Verification items for the finished model (mm, model axes). Face numbers are marked on the shaded views. A direction names the side the tool comes from. Round coordinates to 2 decimals unless told otherwise and drop trailing zeros. Write each loop counter-clockwise with the first axis right and the second up, starting at its lowest first coordinate (ties: lowest second). Pieces come first, ordered by that corner, then holes. Notation, with made-up numbers: (22, -22) - (49, -22) arc R13 ccw to (49, -15) - close; hole circle Ø8 at (41.25, -23.75). An arc over 180 degrees is marked (long way). Answer as a JSON object with one key per item and string values.
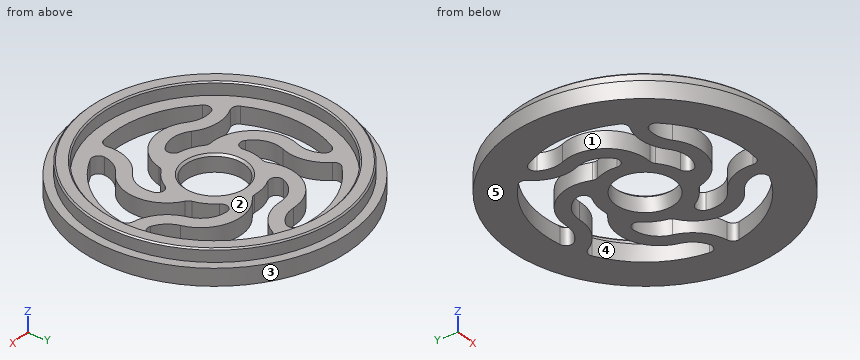
```python
from build123d import *

# Parameters (mm, degrees)
F3_DEPTH = 25.4


with BuildPart() as f1:
    # F0 (on Front) → F1 (revolve)
    with BuildSketch(Plane.XZ):
        Polygon((-25.4, 0), (-5.4737, 0), (-5.4737, 2.794), (-5.8547, 3.175), (-21.3995, 3.175), (-21.3995, 5.334), (-21.6535, 5.588), (-23.5585, 5.588), (-23.8125, 5.334), (-23.8125, 3.175), (-25.4, 3.175), align=None)
    revolve(axis=Axis((0, 0, 7.17671), (0, 0, 1)))

    # F2 (on face) → F3 (cut)
    with BuildSketch(Plane.XY.offset(3.175)):
        with BuildLine():
            ThreePointArc((-7.956627, -0.95471), (-7.931805, 1.142742), (-7.363544, 3.1619))
            ThreePointArc((-7.363544, 3.1619), (-7.260521, 3.657138), (-7.358972, 4.153304))
            ThreePointArc((-7.358972, 4.153304), (-6.561517, 11.480324), (0.065952, 14.704886))
            ThreePointArc((0.065952, 14.704886), (2.327191, 15.1072), (4.180137, 16.464274))
            ThreePointArc((4.180137, 16.464274), (4.415643, 17.713968), (3.449856, 18.541285))
            ThreePointArc((3.449856, 18.541285), (-5.482341, 18.045073), (-13.180977, 13.488609))
            ThreePointArc((-13.180977, 13.488609), (-13.563205, 12.600734), (-13.209763, 11.701011))
            ThreePointArc((-13.209763, 11.701011), (-11.238972, 7.93406), (-11.593134, 3.697492))
            ThreePointArc((-11.593134, 3.697492), (-11.749757, 0.538425), (-10.006841, -2.100984))
            ThreePointArc((-10.006841, -2.100984), (-8.597816, -2.214519), (-7.956627, -0.95471))
        make_face()
        with BuildLine():
            ThreePointArc((-1.55075, -7.862224), (-3.537875, -7.190468), (-5.282606, -6.026065))
            ThreePointArc((-5.282606, -6.026065), (-5.721769, -5.775048), (-6.224075, -5.715357))
            ThreePointArc((-6.224075, -5.715357), (-12.946057, -2.692759), (-13.964798, 4.606784))
            ThreePointArc((-13.964798, 4.606784), (-13.64866, 6.881671), (-14.366722, 9.063287))
            ThreePointArc((-14.366722, 9.063287), (-15.482476, 9.673443), (-16.567745, 9.01058))
            ThreePointArc((-16.567745, 9.01058), (-18.856021, 0.362218), (-16.901576, -8.367645))
            ThreePointArc((-16.901576, -8.367645), (-16.17527, -9.005534), (-15.210364, -8.94742))
            ThreePointArc((-15.210364, -8.94742), (-11.018773, -8.237138), (-7.098999, -9.883138))
            ThreePointArc((-7.098999, -9.883138), (-4.142947, -11.0083), (-1.09413, -10.166311))
            ThreePointArc((-1.09413, -10.166311), (-0.550739, -8.861333), (-1.55075, -7.862224))
        make_face()
        with BuildLine():
            ThreePointArc((-3.366716, 7.272181), (-1.36425, 7.896721), (0.731685, 7.980227))
            ThreePointArc((0.731685, 7.980227), (1.23452, 8.035284), (1.67598, 8.28224))
            ThreePointArc((1.67598, 8.28224), (8.890816, 9.787989), (14.005558, 4.481336))
            ThreePointArc((14.005558, 4.481336), (15.086943, 2.455092), (16.950188, 1.112194))
            ThreePointArc((16.950188, 1.112194), (18.211493, 1.274391), (18.699874, 2.448564))
            ThreePointArc((18.699874, 2.448564), (15.467748, 10.790251), (8.755284, 16.704064))
            ThreePointArc((8.755284, 16.704064), (7.792749, 16.793215), (7.046282, 16.179043))
            ThreePointArc((7.046282, 16.179043), (4.072706, 13.140657), (-0.065952, 12.168314))
            ThreePointArc((-0.065952, 12.168314), (-3.118802, 11.341065), (-5.090438, 8.867832))
            ThreePointArc((-5.090438, 8.867832), (-4.763004, 7.492685), (-3.366716, 7.272181))
        make_face()
        with BuildLine():
            ThreePointArc((5.875882, 5.449165), (7.088652, 3.7377), (7.81575, 1.770152))
            ThreePointArc((7.81575, 1.770152), (8.023497, 1.308941), (8.394785, 0.965402))
            ThreePointArc((8.394785, 0.965402), (12.056344, -5.431014), (8.589959, -11.935269))
            ThreePointArc((8.589959, -11.935269), (6.997053, -13.58987), (6.295656, -15.7769))
            ThreePointArc((6.295656, -15.7769), (6.839679, -16.926351), (8.107302, -17.027989))
            ThreePointArc((8.107302, -17.027989), (15.041935, -11.376332), (18.59204, -3.16493))
            ThreePointArc((18.59204, -3.16493), (18.379389, -2.221956), (17.564605, -1.701813))
            ThreePointArc((17.564605, -1.701813), (13.756043, 0.187313), (11.552374, 3.82294))
            ThreePointArc((11.552374, 3.82294), (9.822231, 6.470739), (6.860777, 7.581605))
            ThreePointArc((6.860777, 7.581605), (5.654118, 6.845253), (5.875882, 5.449165))
        make_face()
        with BuildLine():
            ThreePointArc((6.998211, -3.904412), (5.745278, -5.586696), (4.098714, -6.886213))
            ThreePointArc((4.098714, -6.886213), (3.724274, -7.226314), (3.512283, -7.685589))
            ThreePointArc((3.512283, -7.685589), (-1.439586, -13.14454), (-8.696672, -11.857737))
            ThreePointArc((-8.696672, -11.857737), (-10.762526, -10.854093), (-13.059259, -10.862855))
            ThreePointArc((-13.059259, -10.862855), (-13.984339, -11.735451), (-13.689286, -12.97244))
            ThreePointArc((-13.689286, -12.97244), (-6.171321, -17.82121), (2.735229, -18.660098))
            ThreePointArc((2.735229, -18.660098), (3.566338, -18.166459), (3.809241, -17.230821))
            ThreePointArc((3.809241, -17.230821), (4.428996, -13.024891), (7.205711, -9.805607))
            ThreePointArc((7.205711, -9.805607), (9.189274, -7.341929), (9.330632, -4.182142))
            ThreePointArc((9.330632, -4.182142), (8.257441, -3.262086), (6.998211, -3.904412))
        make_face()
    extrude(amount=-F3_DEPTH, mode=Mode.SUBTRACT)


solid = f1.part
```
Q1. Set-up check for the marked faces 1 and 2: record each of +Z, -Z, +X, -X, +Y, -Y from which the full face is reachable in a straight line by a thin tool's end or side.
Geometry check:
{"face 1": "+Z, -Z", "face 2": "+Z"}
Q2. Material ranges on line 1 along X through (y, z) = (0, 3.75); line 2 along X through (y, z) = (-8, 0.5); line 3 along Y through (x, z) = (2, 1.6), recorded low to high. Write a range as [from, to].
Geometry check:
{"line 1": "x = [-23.81, -21.4], [21.4, 23.81]", "line 2": "x = [-24.11, -17.08], [-1.18, 3.43], [8.89, 11.65], [17.08, 24.11]", "line 3": "y = [-25.32, -18.75], [-10.75, -5.1], [5.1, 8.55], [12.34, 14.98], [18.75, 25.32]"}
Q3. Release check for a two-part mould opening along X. For the marked faces 3, 4 and 5 record: released by +X, released by -X, zero draft, split by the parting line, or undercut.
Geometry check:
{"face 3": "split by the parting line", "face 4": "undercut", "face 5": "zero draft"}
Q4. Section check B-B, the plane z = 4.6. Record the cut outline in (x, y) (1 decimal), then the cut area to 3 significant figures.
Geometry check:
{"outline": "circle Ø47.6 at (0, 0); hole circle Ø42.8 at (0, 0)", "area": "343 mm2"}
Q5. Section check A-A, the plane y = 0. State how many separate pieces and enclosed holes the cut face has, then the cut area to 3 significant figures.
Geometry check:
{"separate pieces": "5", "enclosed holes": "0", "area": "98.3 mm2"}
Q6. Gauge pin test, flat ends, axial feed: P1, Ø15, axis at x = 7, y = -2.5, coming from the +Z side (3 decimals); P2, Ø10, axis at x = 0, y = 0, coming from the -Z side. Record the tip position at first contact, or that the pin passes through.
Geometry check:
{"P1": "stops at z = 3.175", "P2": "passes through"}
